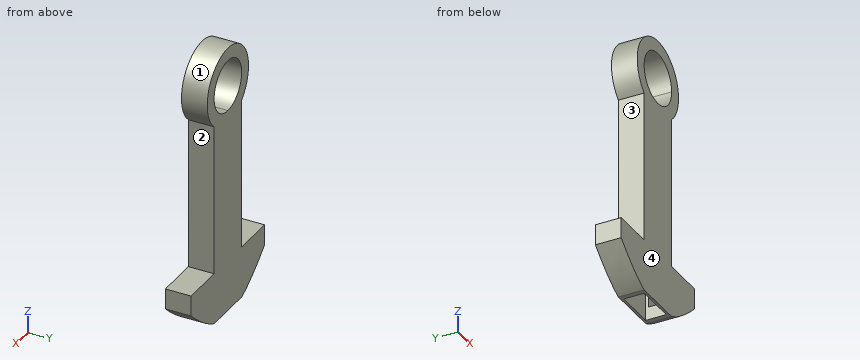
from build123d import *

# Parameters (mm, degrees)
F1_DEPTH      = 12.7
F3_DEPTH      = 19.05
F3_DEPTH_BACK = 19.05
F5_DEPTH      = 12.7


# Not quite as in the source:
# - a feature names something its author has since deleted; it is built from what else it names


with BuildPart() as f1:
    # F0 (on Front) → F1 (new body)
    with BuildSketch(Plane.XZ):
        with BuildLine():
            Line((-12.7, 0), (0, 0))
            Line((0, 0), (12.7, 0))
            Line((12.7, 0), (12.7, 49.3009683429))
            ThreePointArc((12.7, 49.3009683429), (0, 44.45), (-12.7, 49.3009683429))
            Line((-12.7, 49.3009683429), (-12.7, 0))
        make_face()
        Polygon((12.7, 0), (0, 0), (-12.7, 0), (-12.7, -25.4), (0, -25.4), (12.7, -25.4), align=None)
        with BuildLine():
            ThreePointArc((-12.7, 49.3009683429), (0, 44.45), (12.7, 49.3009683429))
            Line((12.7, 49.3009683429), (12.7, 50.8))
            Line((12.7, 50.8), (0, 50.8))
            Line((0, 50.8), (-12.7, 50.8))
            Line((-12.7, 50.8), (-12.7, 49.3009683429))
        make_face()
        with BuildLine():
            Line((12.7, 50.8), (12.7, 49.3009683429))
            ThreePointArc((12.7, 49.3009683429), (17.3901912008, 55.7228700667), (19.05, 63.5))
            ThreePointArc((19.05, 63.5), (13.4703841816, 76.9703841816), (0, 82.55))
            ThreePointArc((0, 82.55), (-17.7959834382, 70.2974608102), (-12.7, 49.3009683429))
            Line((-12.7, 49.3009683429), (-12.7, 50.8))
            Line((-12.7, 50.8), (0, 50.8))
            Line((0, 50.8), (12.7, 50.8))
        make_face()
        with BuildLine():
            ThreePointArc((12.7, 63.5), (8.9802561211, 54.5197438789), (0, 50.8))
            ThreePointArc((0, 50.8), (-8.9802561211, 72.4802561211), (12.7, 63.5))
        make_face(mode=Mode.SUBTRACT)
        with BuildLine():
            Line((33.9128470637, -25.4), (12.7, -25.4))
            Line((12.7, -25.4), (12.7, -50.8))
            add(Edge.make_bspline(
                [(12.7, -50.8), (19.8188597647, -47.7374133591), (26.8761157229, -42.0909685678), (33.9128470637, -35.5836565254)],
                knots=[0.6416254251, 0.6416254251, 0.6416254251, 0.6416254251, 0.8805998947, 0.8805998947, 0.8805998947, 0.8805998947], degree=3))
            Line((33.9128470637, -35.5836565254), (33.9128470637, -25.4))
        make_face()
        Polygon((12.7, -50.8), (12.7, -25.4), (0, -25.4), (-12.7, -25.4), (-12.7, -50.8), align=None)
        with BuildLine():
            Line((-12.7, -50.8), (-12.7, -25.4))
            Line((-12.7, -25.4), (-33.9128470637, -25.4))
            Line((-33.9128470637, -25.4), (-33.9128470637, -35.5836565254))
            add(Edge.make_bspline(
                [(-33.9128470637, -35.5836565254), (-26.8761157229, -42.0909685678), (-19.8188597647, -47.7374133591), (-12.7, -50.8)],
                knots=[0.1194001053, 0.1194001053, 0.1194001053, 0.1194001053, 0.3583745749, 0.3583745749, 0.3583745749, 0.3583745749], degree=3))
        make_face()
    extrude(amount=F1_DEPTH)

    # F2 (on Right) → F3 (cut, two sides)
    with BuildSketch(Plane.YZ) as f3_sk:
        Polygon((-7.62, -31.75), (-10.16, -31.75), (-10.16, -44.45), (-5.08, -44.45), (-2.54, -44.45), (-2.54, -31.75), (-5.08, -31.75), align=None)
    extrude(amount=-F3_DEPTH, mode=Mode.SUBTRACT)
    extrude(f3_sk.sketch, amount=F3_DEPTH_BACK, mode=Mode.SUBTRACT)

    # F4 (on face) → F5 (cut)
    with BuildSketch(Plane(origin=(0, 0, -50.8), x_dir=(1, 0, 0), z_dir=(0, 0, -1))):
        Polygon((-10.1655442268, 1.27), (0, 1.27), (10.16, 1.27), (10.16, 11.43), (0, 11.43), (-10.1655442268, 11.43), align=None)
    extrude(amount=-F5_DEPTH, mode=Mode.SUBTRACT)


solid = f1.part
Work out the finished part from the listing and answer in its coordinate system (mm). Face numbers are marked on the shaded views. A direction names the side the tool comes from. Round coordinates to 2 decimals unless told otherwise and drop trailing zeros. Order: outer loops, then holes, each group sorted by start corner. A loop starts at its lowest first (then second) coordinate and runs counter-clockwise, first axis right, second up. Notation, with made-up numbers: M -2,37 L 51,37 A24 ccw 51,62 Z; hole C 18,76 d5. An arc over 180 degrees is marked long. Put each result on its own line as item: value. Start each with the question number.
Q1. Straight lines are drawn through the part: L1, parallel to X at y = -9.5, z = 63.5; L2, parallel to Z at x = 0, y = -9; L3, parallel to Z at x = 17, y = -2.75. For each, find the intervals that lie inside material, in ascending order. Write a range as [from, to].
Q2. Flat-ended cylindrical pins translate along their axes: pin 1 (6.5 mm diameter, centred on y = -4.5, z = -4.5, fed in from +X); pin 2 (20.5 mm diameter, centred on x = 0, z = 63.5, fed in from +Y); pin 3 (2 mm diameter, centred on y = -8.5, z = -4.5, fed in from -X); pin 4 (5 mm diameter, centred on y = -7.5, z = -45.5, fed in from -X). Find the tip coordinate at first contact, or state that the pin passes through.
Q3. A tool of negligible diameter and unlimited length cuts with its end or side. For the marked faces 1 and 2, from which of +Z, -Z, +X, -X, +Y, -Y can it reach the whole face along a straight path? Write none if from no direction.
Q4. For a pull along Z with two mould halves and no side action, classify the marked faces 3 and 4 as pulls with the +Z half, pulls with the -Z half, needs draft (parallel to the pull), parting line crosses it, or undercut.
Q5. Section B-B, the plane z = -10.5 is taken. Write down the section's boundary in (x, y), and give its area (3 significant figures).
Q6. Section A-A, the plane z = 65.5 is taken. Write down the section's boundary in (x, y), and give its area (3 significant figures).
Findings below:
1. L1: x = [-19.05, -12.7], [12.7, 19.05]
1. L2: z = [-31.75, 50.8], [76.2, 82.55]
1. L3: z = [-48.65, -44.45], [-31.75, -25.4], [54.9, 72.1]
2. pin 1: stops at x = 12.7
2. pin 2: passes through
2. pin 3: stops at x = -12.7
2. pin 4: stops at x = -25.29
3. face 1: +Y, -Y
3. face 2: +X, +Y, -Y
4. face 3: undercut
4. face 4: needs draft
5. outline: M -12.7,-12.7 L 12.7,-12.7 L 12.7,0 L -12.7,0 Z
5. area: 323 mm^2
6. outline: M -18.94,-12.7 L -12.54,-12.7 L -12.54,0 L -18.94,0 Z; M 12.54,-12.7 L 18.94,-12.7 L 18.94,0 L 12.54,0 Z
6. area: 163 mm^2
